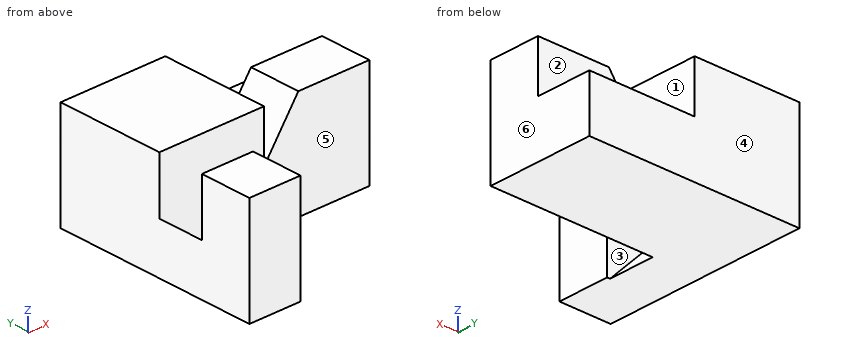
from build123d import *

# Parameters (mm, degrees)
F0_W     = 15.748
F0_H     = 15.748
F1_DEPTH = 15.9512
F3_DEPTH = 6.8834
F5_DEPTH = 7.6708
F6_W     = 15.9512
F6_H     = 8.2042
F7_DEPTH = 15.8496
F9_DEPTH = 7.6454


with BuildPart() as f1:
    # F0 (on Front) → F1 (new body)
    with BuildSketch(Plane.XZ):
        with Locations((7.874, 7.874)):
            Rectangle(F0_W, F0_H)
    extrude(amount=F1_DEPTH)

    # F2 (on face) → F3 (join)
    with BuildSketch(Plane.XZ.offset(15.9512)):
        Polygon((0, 7.4676), (0, 0), (7.239, 0), align=None)
    extrude(amount=F3_DEPTH)

    # F4 (on face) → F5 (join)
    with BuildSketch(Plane.XZ.offset(22.8346)):
        Polygon((0, 7.4676), (7.239, 0), (7.6962, 0), (7.6962, 15.748), (0, 15.748), align=None)
        Polygon((0, 7.4676), (0, 0), (7.239, 0), align=None)
    extrude(amount=F5_DEPTH)

    # F6 (on face) → F7 (join)
    with BuildSketch(Plane.YZ.offset(15.748)):
        with Locations((-7.9756, 4.1021)):
            Rectangle(F6_W, F6_H)
    extrude(amount=F7_DEPTH)

    # F8 (on face) → F9 (join)
    with BuildSketch(Plane.XZ.offset(15.9512)):
        Polygon((20.9155736628, 15.748), (15.748, 8.2042), (31.5976, 8.2042), (31.5976, 15.748), align=None)
    extrude(amount=-F9_DEPTH)


solid = f1.part
Geometry check sheet. Reference: the model listing, model coordinates, mm. Face numbers are marked on the shaded views. A direction names the side the tool comes from. Coordinates: 2 decimals unless noted, no trailing zeros. Order: outer loops, then holes, each group sorted by start corner. A loop starts at its lowest first (then second) coordinate and runs counter-clockwise, first axis right, second up. Notation, with made-up numbers: M 36,87.25 L 46,87.25 A20 cw 46,120.25 Z; hole C -14,-25.5 d10. An arc over 180 degrees is marked long. Use CSV: the item, a comma, the result in double quotes.
Item 1: Gauge pin test, flat ends, axial feed: pin 1 Ø4 at (y, z) = (-26.5, 6.5) entering from +X; pin 2 Ø9 at (x, y) = (27, -3.5) entering from +Z; pin 3 Ø4.5 at (x, z) = (15.5, 8) entering from -Y; pin 4 Ø1 at (y, z) = (-16.5, 13) entering from +X. Record the tip position at first contact, or that the pin passes through.
Returned:
pin 1,"stops at x = 7.7"
pin 2,"stops at z = 8.2"
pin 3,"stops at y = -15.95"
pin 4,"passes through"
Item 2: Cross-section at A-A on z = 9.5. Record the cut outline in (x, y).
Returned:
outline,"M 0,-30.51 L 7.7,-30.51 L 7.7,-22.83 L 0,-22.83 Z; M 0,-15.95 L 15.75,-15.95 L 15.75,0 L 0,0 Z; M 16.64,-15.95 L 31.6,-15.95 L 31.6,-8.31 L 16.64,-8.31 Z"
Item 3: Cross-section at C-C on x = 24. Record the cut outline in (y, z).
Returned:
outline,"M -15.95,0 L 0,0 L 0,8.2 L -8.31,8.2 L -8.31,15.75 L -15.95,15.75 Z"
Item 4: Tool access check on the marked faces 1, 2 and 3. Record the directions out of +Z, -Z, +X, -X, +Y, -Y that give a thin tool (end or side, any length) a straight path to the whole face; none if there is none.
Returned:
face 1,"+Z, +Y, -Y"
face 2,"+Z, +X, +Y"
face 3,"+Z, +X"
Item 5: Mould release check, pull along Y, two halves, no side actions. Record for the marked faces 4, 5 and 6: pulls with the +Y half, pulls with the -Y half, needs draft (parallel to the pull), parting line crosses it, or undercut.
Returned:
face 4,"pulls with the +Y half"
face 5,"undercut"
face 6,"needs draft"
Item 6: Thickness scan on line 1 along Y through (x, z) = (5, 13.25); line 2 along Y through (x, z) = (25.5, 10.75); line 3 along X through (y, z) = (-6, 8.75). Record the ranges inside material, lowest first.
Returned:
line 1,"y = -30.51 to -22.83, -15.95 to 0"
line 2,"y = -15.95 to -8.31"
line 3,"x = 0 to 15.75"
Item 7: Cross-section at D-D on z = 14. Record the cut outline in (x, y).
Returned:
outline,"M 0,-30.51 L 7.7,-30.51 L 7.7,-22.83 L 0,-22.83 Z; M 0,-15.95 L 15.75,-15.95 L 15.75,0 L 0,0 Z; M 19.72,-15.95 L 31.6,-15.95 L 31.6,-8.31 L 19.72,-8.31 Z"
Item 8: Cross-section at B-B on y = -7. Record the cut outline in (x, z), then the cut area to 3 significant figures.
Returned:
outline,"M 0,0 L 31.6,0 L 31.6,8.2 L 15.75,8.2 L 15.75,15.75 L 0,15.75 Z"
area,"378 mm2"
